Input: part model. Units: mm. Frame: model coordinates. A direction names the side the tool comes from. Give positions to 0.01 mm unless a question says otherwise; leave off trailing zeros. Loops run counter-clockwise (first coordinate to the right, second up) from the corner with the lowest first, then second, coordinate; pieces in that order, holes last. Notation, with made-up numbers: M 64,59.5 L 84,59.5 A30 cw 84,87.5 Z; hole C -37,26.5 d4. An arc over 180 degrees is marked long. Answer as a JSON object with one key per item and string values. Group by question number.
1) Ray query, L1, parallel to X at y = 1.7, z = -10.5; L2, parallel to Z at x = -7.75, y = 0.5; L3, parallel to Z at x = 13, y = 0.9. Return the intervals inside material, ascending.
2) Section query C-C on z = 40. Return loops of the section in (x, y), plus the area to 3 significant figures.
3) Section query B-B on x = -3.25. Return loops of the section in (y, z).
4) First-contact query: P1, Ø0.9, axis at x = 1, y = 2, coming from the +Z side; P2, Ø1.5, axis at y = 1.5, z = -2.5, coming from the -X side; P3, Ø11.5, axis at x = 10.5, z = -27.45, coming from the -Y side; P4, Ø1.1, axis at x = 6.5, y = 1.5, coming from the +Z side. Flat tips, straight axial feed; report the tip coordinate or a pass-through.
5) Section query D-D on y = 1.5. Count the separate pieces of the cut face and the enclosed holes in it, plus the area to 3 significant figures.
6) Access query for faces 1 (the flat face through (18.5, 1, 0)), 2 (the flat face through (-6, 1, -9)), 3 (the flat face through (-8, 1, 7.5)). Directions: +Z, -Z, +X, -X, +Y, -Y. A direction counts if a zero-diameter tool reaches every point of the face in a straight line with its end or side. Return the directions, or none.
7) Draft query along Z for faces 4 (the flat face through (7.2, 0, -0.6)), 5 (the cylindrical face through (17.81, 1.48, -30.7)), 6 (the cylindrical face through (-5.394, 1.479, 45.714)), 7 (the flat face through (6, 1, 9)). Return one class per face: +Z half, -Z half, draft (parallel to the pull), parting line (faces both ways), or undercut.
8) Section query A-A on x = 10.5. Return loops of the section in (y, z), plus the area to 3 significant figures.
from build123d import *

# Parameters (mm, degrees)
SKETCH1_R           = 4.5
SKETCH1_R_2         = 1.5
BOSS_EXTRUDE1_DEPTH = 3
BOSS_EXTRUDE2_START = -3
SKETCH3_R           = 4.5
SKETCH3_R_2         = 4
BOSS_EXTRUDE2_DEPTH = 3


with BuildPart() as part:
    # Sketch1 → Boss-Extrude1 (new body)
    with BuildSketch(Plane(origin=(0, 0, 0), x_dir=(1, 0, 0), z_dir=(0, 1, 0))):
        with BuildLine():
            Line((-6, -7.5), (-10, -7.5))
            Line((-10, -7.5), (-10, -8.75))
            Line((-10, -8.75), (-10, -38.449422848))
            ThreePointArc((-10, -38.449422848), (-5.277416427, -45.767940555), (3.336657191, -44.479052382))
            Line((3.336657191, -44.479052382), (15.796770322, -33.445350211))
            ThreePointArc((15.796770322, -33.445350211), (17.792942369, -30.73831136), (18.5, -27.450024315))
            Line((18.5, -27.450024315), (18.5, 27.45))
            ThreePointArc((18.5, 27.45), (17.789725141, 30.745437355), (15.785023159, 33.455708135))
            Line((15.785023159, 33.455708135), (3.285023159, 44.455708135))
            ThreePointArc((3.285023159, 44.455708135), (-5.295437355, 45.739725141), (-10, 38.45))
            Line((-10, 38.45), (-10, 8.75))
            Line((-10, 8.75), (-10, 7.5))
            Line((-10, 7.5), (-6, 7.5))
            Line((-6, 7.5), (-6, 10.5))
            Line((-6, 10.5), (-4.571851993, 11.5))
            Line((-4.571851993, 11.5), (4.571851993, 11.5))
            Line((4.571851993, 11.5), (6, 10.5))
            Line((6, 10.5), (6, 7.5))
            Line((6, 7.5), (7, 7.5))
            Line((7, 7.5), (7, 0))
            Line((7, 0), (7, -7.5))
            Line((7, -7.5), (6, -7.5))
            Line((6, -7.5), (6, -10.5))
            Line((6, -10.5), (4.571851993, -11.5))
            Line((4.571851993, -11.5), (-4.571851993, -11.5))
            Line((-4.571851993, -11.5), (-6, -10.5))
            Line((-6, -10.5), (-6, -7.5))
        make_face()
        with Locations(Location((-2, -38.45, 0), (0, 0, 270))):
            Circle(SKETCH1_R, mode=Mode.SUBTRACT)
        with Locations(Location((-6.57936952, -14.367032155, 0), (0, 0, 270))):
            Circle(SKETCH1_R_2, mode=Mode.SUBTRACT)
        with Locations(Location((10.5, -27.45, 0), (0, 0, 270))):
            Circle(SKETCH1_R, mode=Mode.SUBTRACT)
        with Locations(Location((6.57936952, -14.367032155, 0), (0, 0, 270))):
            Circle(SKETCH1_R_2, mode=Mode.SUBTRACT)
        with Locations(Location((-6.57936952, 14.367032155, 0), (0, 0, 270))):
            Circle(SKETCH1_R_2, mode=Mode.SUBTRACT)
        with Locations(Location((-2, 38.45, 0), (0, 0, 270))):
            Circle(SKETCH1_R, mode=Mode.SUBTRACT)
        with Locations(Location((6.57936952, 14.367032155, 0), (0, 0, 270))):
            Circle(SKETCH1_R_2, mode=Mode.SUBTRACT)
        with Locations(Location((10.5, 27.45, 0), (0, 0, 270))):
            Circle(SKETCH1_R, mode=Mode.SUBTRACT)
    extrude(amount=BOSS_EXTRUDE1_DEPTH)

    # Sketch3 → Boss-Extrude2 (add)
    # profile 1 of 2: a face of its own
    with BuildSketch(Plane(origin=(0, 3, 0), x_dir=(1, 0, 0), z_dir=(0, 1, 0)).offset(BOSS_EXTRUDE2_START)):
        with Locations((-2, -38.45)):
            Circle(SKETCH3_R)
        with Locations(Location((-2, -38.45, 0), (0, 0, 270))):
            Circle(SKETCH3_R_2, mode=Mode.SUBTRACT)
    # profile 2 of 2: a face of its own
    with BuildSketch(Plane(origin=(0, 3, 0), x_dir=(1, 0, 0), z_dir=(0, 1, 0)).offset(BOSS_EXTRUDE2_START)):
        with Locations((10.5, -27.45)):
            Circle(SKETCH3_R)
        with Locations(Location((10.5, -27.45, 0), (0, 0, 270))):
            Circle(SKETCH3_R_2, mode=Mode.SUBTRACT)
    extrude(amount=BOSS_EXTRUDE2_DEPTH)


solid = part.part
Output:
{
 "1": {"L1": "x = -10 to -6, 6 to 18.5", "L2": "z = -44.01 to -15.3, -13.43 to -7.5, 7.5 to 13.43, 15.3 to 44.02", "L3": "z = -35.91 to -31.19, -23.71 to 24.33, 30.57 to 35.92"},
 "2": {"outline": "M -9.85,0 L -5.69,0 L -5.69,3 L -9.85,3 Z; M 1.69,0 L 8.39,0 L 8.39,3 L 1.69,3 Z", "area": "32.6 mm^2"},
 "3": {"outline": "M 0,-46.35 L 3,-46.35 L 3,-42.77 L 0,-42.77 Z; M 0,-34.13 L 3,-34.13 L 3,-11.5 L 0,-11.5 Z; M 0,11.5 L 3,11.5 L 3,34.65 L 0,34.65 Z; M 0,42.25 L 3,42.25 L 3,46.38 L 0,46.38 Z"},
 "4": {"P1": "stops at z = 46.08", "P2": "stops at x = 7", "P3": "stops at y = 0", "P4": "stops at z = 42.16"},
 "5": {"separate pieces": "1", "enclosed holes": "8", "area": "1,740 mm^2"},
 "6": {"face 1": "+Z, -Z, +X, +Y, -Y", "face 2": "+Y, -Y", "face 3": "-X, +Y, -Y"},
 "7": {"face 4": "draft", "face 5": "-Z half", "face 6": "+Z half", "face 7": "undercut"},
 "8": {"outline": "M 0,-38.11 L 3,-38.11 L 3,-31.95 L 0,-31.95 Z; M 0,-22.95 L 3,-22.95 L 3,23.45 L 0,23.45 Z; M 0,31.45 L 3,31.45 L 3,38.14 L 0,38.14 Z", "area": "178 mm^2"}
}
